Build history of the part. All positions in model axes, mm. Face numbers are marked on the shaded views. A direction names the side the tool comes from. Give positions to 0.01 mm unless a question says otherwise; leave off trailing zeros. Order: outer loops, then holes, each group sorted by start corner. A loop starts at its lowest first (then second) coordinate and runs counter-clockwise, first axis right, second up. Notation, with made-up numbers: M 82.5,9.5 L 141.5,9.5 A35 cw 141.5,48.5 Z; hole C 24.25,-15.75 d8. An arc over 180 degrees is marked long. One line per item, written item: value.
from build123d import *

# Parameters (mm, degrees)
SKETCH1_R                                       = 6
BOSS_EXTRUDE1_DEPTH                             = 3.9
SKETCH5_R                                       = 8
SKETCH5_R_2                                     = 2.05
SKETCH5_R_3                                     = 0.525
BOSS_EXTRUDE3_DEPTH                             = 0.5
CSK_FOR_M2_FLAT_HEAD_MACHINE_SCREW1_D           = 2.6
CSK_FOR_M2_FLAT_HEAD_MACHINE_SCREW1_CSINK_D     = 4.4
CSK_FOR_M2_FLAT_HEAD_MACHINE_SCREW1_CSINK_ANGLE = 90


with BuildPart() as part:
    # Sketch1 → Boss-Extrude1 (new body)
    with BuildSketch(Plane.XY):
        with BuildLine():
            Line((-2.5, -12.951833847), (-2.5, -38.5))
            Line((-2.5, -38.5), (2.5, -38.5))
            Line((2.5, -38.5), (2.5, -12.951833847))
            ThreePointArc((2.5, -12.951833847), (3.295532486, -9.043154047), (5.555555556, -5.756370599))
            ThreePointArc((5.555555556, -5.756370599), (0, 8), (-5.555555556, -5.756370599))
            ThreePointArc((-5.555555556, -5.756370599), (-3.295532486, -9.043154047), (-2.5, -12.951833847))
        make_face()
        Circle(SKETCH1_R, mode=Mode.SUBTRACT)
    extrude(amount=BOSS_EXTRUDE1_DEPTH)

    # Sketch5 → Boss-Extrude3 (add)
    with BuildSketch(Plane(origin=(0, 0, 0), x_dir=(-1, 0, 0), z_dir=(0, 0, -1))):
        Circle(SKETCH5_R)
        Circle(SKETCH5_R_2, mode=Mode.SUBTRACT)
        with Locations((4.2, 0)):
            Circle(SKETCH5_R_3, mode=Mode.SUBTRACT)
        with Locations((-4.2, 0)):
            Circle(SKETCH5_R_3, mode=Mode.SUBTRACT)
    extrude(amount=-BOSS_EXTRUDE3_DEPTH)

    # CSK for M2 Flat Head Machine Screw1 (through all)
    with Locations(Plane(origin=(0, 0, 0), x_dir=(-1, 0, 0), z_dir=(0, 0, -1))):
        with Locations((0, -33.5), (0, -23.5)):
            CounterSinkHole(CSK_FOR_M2_FLAT_HEAD_MACHINE_SCREW1_D / 2, CSK_FOR_M2_FLAT_HEAD_MACHINE_SCREW1_CSINK_D / 2, counter_sink_angle=CSK_FOR_M2_FLAT_HEAD_MACHINE_SCREW1_CSINK_ANGLE)


solid = part.part
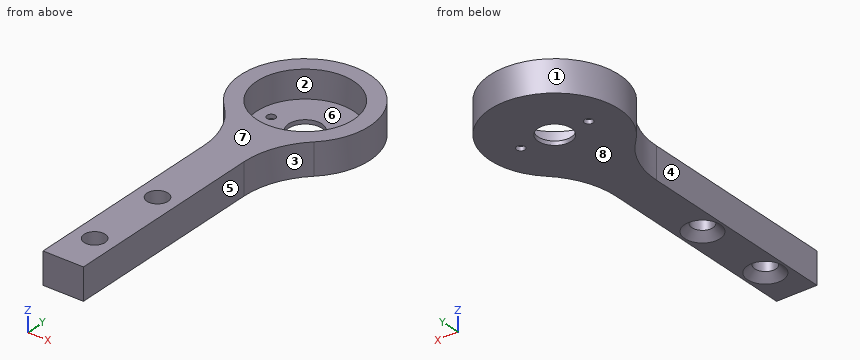
1) Saw through at D-D, the plane y = -33.5. Write the cut outline in (x, z).
Check values:
outline: M -2.5,0 L -2.2,0 L -1.3,0.9 L -1.3,3.9 L -2.5,3.9 Z; M 1.3,0.9 L 2.2,0 L 2.5,0 L 2.5,3.9 L 1.3,3.9 Z
2) Tool access for the marked faces 4, 5, 6, 7 and 8: list every direction of +Z, -Z, +X, -X, +Y, -Y with a clear straight run to the whole face (end or side of a thin tool).
Check values:
face 4: +Z, -Z, -X, -Y
face 5: +Z, -Z, +X, -Y
face 6: +Z
face 7: +Z, +X, -X, +Y, -Y
face 8: -Z, +X, -X, +Y, -Y
3) Saw through at C-C, the plane x = 0. Write the cut outline in (y, z), then the cut area to 3 significant figures.
Check values:
outline: M -38.5,0 L -35.7,0 L -34.8,0.9 L -34.8,3.9 L -38.5,3.9 Z; M -32.2,0.9 L -31.3,0 L -25.7,0 L -24.8,0.9 L -24.8,3.9 L -32.2,3.9 Z; M -22.2,0.9 L -21.3,0 L -2.05,0 L -2.05,0.5 L -6,0.5 L -6,3.9 L -22.2,3.9 Z; M 2.05,0 L 8,0 L 8,3.9 L 6,3.9 L 6,0.5 L 2.05,0.5 Z
area: 117 mm^2
4) Pin check, flat tips, straight feed: pin 1 (2.5 mm diameter, centred on x = 0, y = 0, fed in from -Z); pin 2 (3 mm diameter, centred on x = 3.5, y = 0, fed in from +Z); pin 3 (1.2 mm diameter, centred on y = -24.5, z = 2, fed in from -X); pin 4 (2 mm diameter, centred on y = -29, z = 1, fed in from +X). Stop position of each tip, or through.
Check values:
pin 1: through
pin 2: z = 0.5
pin 3: x = -2.5
pin 4: x = 2.5
5) Saw through at B-B, the plane z = 2.55. Write the cut outline in (x, y), then the cut area to 3 significant figures.
Check values:
outline: M -5.56,-5.76 A10 cw -2.5,-12.95 L -2.5,-38.5 L 2.5,-38.5 L 2.5,-12.95 A10 cw 5.56,-5.76 A8 ccw long Z; hole C 0,0 d12; hole C 0,-33.5 d2.6; hole C 0,-23.5 d2.6
area: 238 mm^2
6) Drill centre lines: probe 1 along Y at (x, z) = (0, 1.8); probe 2 along X at (y, z) = (0, 3.5); probe 3 along Y at (x, z) = (0, 0.25). Where is each one in solid material? Low to high. Write a range as from..to.
Check values:
probe 1: -38.5..-34.8, -32.2..-24.8, -22.2..-6, 6..8
probe 2: -8..-6, 6..8
probe 3: -38.5..-35.45, -31.55..-25.45, -21.55..-2.05, 2.05..8
7) Saw through at A-A, the plane y = 0. Write the cut outline in (x, z) (3 decimals), then the cut area to 3 significant figures.
Check values:
outline: M -8,0 L -4.725,0 L -4.725,0.5 L -6,0.5 L -6,3.9 L -8,3.9 Z; M -3.675,0 L -2.05,0 L -2.05,0.5 L -3.675,0.5 Z; M 2.05,0 L 3.675,0 L 3.675,0.5 L 2.05,0.5 Z; M 4.725,0 L 8,0 L 8,3.9 L 6,3.9 L 6,0.5 L 4.725,0.5 Z
area: 18.5 mm^2
8) Mould opens along X. For the marked faces 1, 2 and 3 say: released by +X, released by -X, zero draft, split by the parting line, or undercut.
Check values:
face 1: split by the parting line
face 2: undercut
face 3: released by +X
